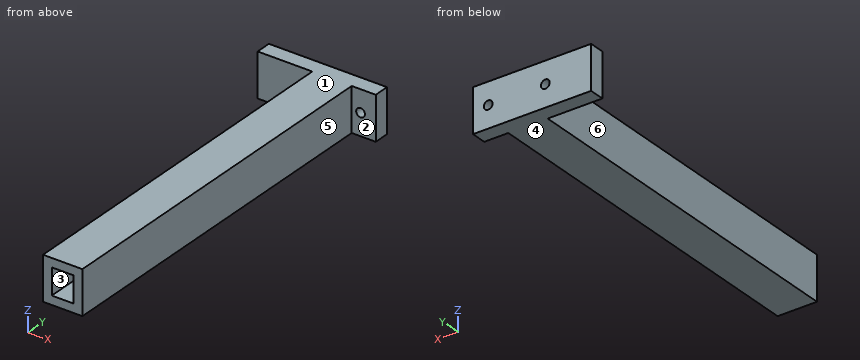
```python
from build123d import *

# Parameters (mm, degrees)
SKETCH1_W           = 40
SKETCH1_H           = 20
BOSS_EXTRUDE1_DEPTH = 7
SKETCH2_R           = 2
CUT_EXTRUDE1_DEPTH  = 25.19584861
SKETCH3_W           = 18
SKETCH3_H           = 20
BOSS_EXTRUDE2_DEPTH = 167.64
SKETCH4_W           = 10
SKETCH4_H           = 12
CUT_EXTRUDE2_DEPTH  = 167.64
SKETCH7_W           = 20
SKETCH7_H           = 7
BOSS_EXTRUDE3_DEPTH = 14


with BuildPart() as part:
    # Sketch1 → Boss-Extrude1 (new body)
    with BuildSketch(Plane(origin=(0, 0, 0), x_dir=(1, 0, 0), z_dir=(0, 1, 0))):
        with Locations((0.745622296, 0.298458403)):
            Rectangle(SKETCH1_W, SKETCH1_H)
    extrude(amount=BOSS_EXTRUDE1_DEPTH)

    # Sketch2 → Cut-Extrude1 (cut, through all)
    with BuildSketch(Plane(origin=(0, 7, 0), x_dir=(1, 0, 0), z_dir=(0, 1, 0))):
        with Locations(Location((-12.304377704, 0.298458403, 0), (0, 0, 270))):
            Circle(SKETCH2_R)
        with Locations(Location((13.795622296, 0.298458403, 0), (0, 0, 270))):
            Circle(SKETCH2_R)
    extrude(amount=-CUT_EXTRUDE1_DEPTH, mode=Mode.SUBTRACT)

    # Sketch3 → Boss-Extrude2 (add)
    with BuildSketch(Plane(origin=(0, 0, 0), x_dir=(-1, 0, 0), z_dir=(0, -1, 0))):
        with Locations((-0.745622296, 0.298458403)):
            Rectangle(SKETCH3_W, SKETCH3_H)
    extrude(amount=BOSS_EXTRUDE2_DEPTH)

    # Sketch4 → Cut-Extrude2 (cut)
    with BuildSketch(Plane.XZ.offset(167.64)):
        with Locations((0.745622296, -0.298458403)):
            Rectangle(SKETCH4_W, SKETCH4_H)
    extrude(amount=-CUT_EXTRUDE2_DEPTH, mode=Mode.SUBTRACT)

    # Sketch7 → Boss-Extrude3 (add)
    with BuildSketch(Plane.ZY.offset(19.254377704)):
        with Locations((-0.298458403, 3.5)):
            Rectangle(SKETCH7_W, SKETCH7_H)
    extrude(amount=BOSS_EXTRUDE3_DEPTH)


solid = part.part
```
Model file for the job. Use its own axes, mm. Face numbers are marked on the shaded views. A direction names the side the tool comes from. Give positions to 0.01 mm unless a question says otherwise; leave off trailing zeros. Loops run counter-clockwise (first coordinate to the right, second up) from the corner with the lowest first, then second, coordinate; pieces in that order, holes last. Notation, with made-up numbers: M -21.5,-30 L 18.5,-30 A6 ccw 18.5,-20 Z; hole C 74.25,-39 d6. An arc over 180 degrees is marked long. Use one line per item in the form item = value.
Item 1: Slice it at A-A on y = -155. List the corners of the cut face in (x, z).
Filled in:
outline = M -8.25,-10.3 L 9.75,-10.3 L 9.75,9.7 L -8.25,9.7 Z; hole M -4.25,-6.3 L 5.75,-6.3 L 5.75,5.7 L -4.25,5.7 Z
Item 2: Two-plate mould, pull along Z, no slides. Class the marked faces 1, 2 and 3: released by +Z, released by -Z, zero draft, split by the parting line, or undercut.
Filled in:
face_1 = released by +Z
face_2 = zero draft
face_3 = undercut
Item 3: Which spindle directions (+Z, -Z, +X, -X, +Y, -Y) get a long thin tool onto all of the face, cutting with end or side? Do the marked faces 4, 5 and 6. Say none if no direction does.
Filled in:
face_4 = -Z, +X, -X, +Y, -Y
face_5 = +Z, -Z, +X, -Y
face_6 = +Z, -Z, -X, -Y
Item 4: Flat gauge pins, fed straight in: pin 1 Ø3 at (y, z) = (-32, -6) entering from -X; pin 2 Ø6 at (x, z) = (11.5, -7) entering from -Y; pin 3 Ø8 at (y, z) = (-76, -6) entering from +X; pin 4 Ø10 at (x, z) = (-16, 3) entering from -Y. Where does each tip first touch, or does it go through?
Filled in:
pin_1 = -8.25
pin_2 = -167.64
pin_3 = 9.75
pin_4 = 0
Item 5: Drill centre lines: L1, parallel to X at y = -119, z = 1.5; L2, parallel to Z at x = 4.5, y = -97; L3, parallel to X at y = -23, z = 6. Where is each one in solid material? Low to high.
Filled in:
L1 = -8.25 to -4.25, 5.75 to 9.75
L2 = -10.3 to -6.3, 5.7 to 9.7
L3 = -8.25 to 9.75
Item 6: Slice it at D-D on x = -22. List the corners of the cut face in (y, z), and give its area (3 significant figures).
Filled in:
outline = M 0,-10.3 L 7,-10.3 L 7,9.7 L 0,9.7 Z
area = 140 mm^2
Item 7: Slice it at C-C on z = -0.5. List the corners of the cut face in (x, y).
Filled in:
outline = M -33.25,0 L -14.29,0 L -14.29,7 L -33.25,7 Z; M -10.31,0 L -8.25,0 L -8.25,-167.64 L -4.25,-167.64 L -4.25,0 L 5.75,0 L 5.75,-167.64 L 9.75,-167.64 L 9.75,0 L 11.81,0 L 11.81,7 L -10.31,7 Z; M 15.79,0 L 20.75,0 L 20.75,7 L 15.79,7 Z
Item 8: Slice it at B-B on x = 0.5. List the corners of the cut face in (y, z).
Filled in:
outline = M -167.64,-10.3 L 7,-10.3 L 7,9.7 L -167.64,9.7 L -167.64,5.7 L 0,5.7 L 0,-6.3 L -167.64,-6.3 Z
